CAD build for the part. Positions are in the model's coordinates, mm. A direction names the side the tool comes from. Coordinates: 2 decimals unless noted, no trailing zeros. Write each loop counter-clockwise with the first axis right and the second up, starting at its lowest first coordinate (ties: lowest second). Pieces come first, ordered by that corner, then holes. Notation, with made-up numbers: (-3, -32) -> (16, -32) arc R30 ccw to (16, -6) -> close; hole circle Ø8 at (18.5, 32.5). An arc over 180 degrees is marked (long way). Answer as CSV lines item,"result". Start each with the question number.
```python
from build123d import *

# Parameters (mm, degrees)
SKIZZE1_W                       = 60
SKIZZE1_H                       = 72.2
AUFSATZ_LINEAR_AUSTRAGEN1_DEPTH = 4
AUFSATZ_LINEAR_START            = -6
SKIZZE2_W                       = 60
SKIZZE2_H                       = 3
AUFSATZ_LINEAR_AUSTRAGEN2_DEPTH = 10
SKIZZE4_R                       = 2
SCHNITT_LINEAR_AUSTRAGEN1_DEPTH = 51.287274732
F_LLMUSTER1_OUTLINE_R           = 2
F_LLMUSTER1_DEPTH               = 4


# Read off the part's stored shape, not the designer's step: Füllmuster1
with BuildPart() as part:
    # Skizze1 → Aufsatz-Linear austragen1 (new body)
    with BuildSketch(Plane(origin=(0, 0, 0), x_dir=(1, 0, 0), z_dir=(0, 1, 0))):
        Rectangle(SKIZZE1_W, SKIZZE1_H)
    extrude(amount=AUFSATZ_LINEAR_AUSTRAGEN1_DEPTH)

    # Skizze2 → Aufsatz-Linear austragen2 (add)
    with BuildSketch(Plane(origin=(0, 0, 0), x_dir=(1, 0, 0), z_dir=(0, 1, 0)).offset(AUFSATZ_LINEAR_START)):
        with Locations((0, 37.6)):
            Rectangle(SKIZZE2_W, SKIZZE2_H)
    aufsatz_linear_austragen2 = extrude(amount=AUFSATZ_LINEAR_AUSTRAGEN2_DEPTH)

    # Spiegeln1: Aufsatz-Linear austragen2 across plane
    add(aufsatz_linear_austragen2.mirror(Plane.XY))

    # Skizze4 → Schnitt-Linear austragen1 (cut, through all)
    with BuildSketch(Plane(origin=(0, 4, 0), x_dir=(1, 0, 0), z_dir=(0, 1, 0))):
        with Locations(Location((0, 0, 0), (0, 0, 270))):
            Circle(SKIZZE4_R)
    extrude(amount=-SCHNITT_LINEAR_AUSTRAGEN1_DEPTH, mode=Mode.SUBTRACT)

    # Füllmuster1 outline → Füllmuster1 (cut)
    with BuildSketch(Plane(origin=(0, 0, 0), x_dir=(1, 0, 0), z_dir=(0, 1, 0))):
        with Locations((6.3, 0)):
            Circle(F_LLMUSTER1_OUTLINE_R)
        with Locations((17.760190533, 6.464180709)):
            Circle(F_LLMUSTER1_OUTLINE_R)
        with Locations((14.478239975, 12.148685823)):
            Circle(F_LLMUSTER1_OUTLINE_R)
        with Locations((9.45, 16.367880132)):
            Circle(F_LLMUSTER1_OUTLINE_R)
        with Locations((6.3, 10.911920088)):
            Circle(F_LLMUSTER1_OUTLINE_R)
        with Locations((0, 12.6)):
            Circle(F_LLMUSTER1_OUTLINE_R)
        with Locations((-6.3, 10.911920088)):
            Circle(F_LLMUSTER1_OUTLINE_R)
        with Locations((-10.911920088, 6.3)):
            Circle(F_LLMUSTER1_OUTLINE_R)
        with Locations((-12.6, 0)):
            Circle(F_LLMUSTER1_OUTLINE_R)
        with Locations((-10.911920088, -6.3)):
            Circle(F_LLMUSTER1_OUTLINE_R)
        with Locations((-6.3, -10.911920088)):
            Circle(F_LLMUSTER1_OUTLINE_R)
        with Locations((0, -12.6)):
            Circle(F_LLMUSTER1_OUTLINE_R)
        with Locations((3.15, -5.455960044)):
            Circle(F_LLMUSTER1_OUTLINE_R)
        with Locations((-3.15, -5.455960044)):
            Circle(F_LLMUSTER1_OUTLINE_R)
        with Locations((-6.3, 0)):
            Circle(F_LLMUSTER1_OUTLINE_R)
        with Locations((-3.15, 5.455960044)):
            Circle(F_LLMUSTER1_OUTLINE_R)
        with Locations((3.15, 5.455960044)):
            Circle(F_LLMUSTER1_OUTLINE_R)
        with Locations((12.6, 0)):
            Circle(F_LLMUSTER1_OUTLINE_R)
        with Locations((10.911920088, -6.3)):
            Circle(F_LLMUSTER1_OUTLINE_R)
        with Locations((6.3, -10.911920088)):
            Circle(F_LLMUSTER1_OUTLINE_R)
        with Locations((3.281950558, 18.612866532)):
            Circle(F_LLMUSTER1_OUTLINE_R)
        with Locations((-3.281950558, 18.612866532)):
            Circle(F_LLMUSTER1_OUTLINE_R)
        with Locations((-9.45, 16.367880132)):
            Circle(F_LLMUSTER1_OUTLINE_R)
        with Locations((-14.478239975, 12.148685823)):
            Circle(F_LLMUSTER1_OUTLINE_R)
        with Locations((-17.760190533, 6.464180709)):
            Circle(F_LLMUSTER1_OUTLINE_R)
        with Locations((-18.9, 0)):
            Circle(F_LLMUSTER1_OUTLINE_R)
        with Locations((-17.760190533, -6.464180709)):
            Circle(F_LLMUSTER1_OUTLINE_R)
        with Locations((-14.478239975, -12.148685823)):
            Circle(F_LLMUSTER1_OUTLINE_R)
        with Locations((-9.45, -16.367880132)):
            Circle(F_LLMUSTER1_OUTLINE_R)
        with Locations((-3.281950558, -18.612866532)):
            Circle(F_LLMUSTER1_OUTLINE_R)
        with Locations((3.281950558, -18.612866532)):
            Circle(F_LLMUSTER1_OUTLINE_R)
        with Locations((9.45, -16.367880132)):
            Circle(F_LLMUSTER1_OUTLINE_R)
        with Locations((14.478239975, -12.148685823)):
            Circle(F_LLMUSTER1_OUTLINE_R)
        with Locations((17.760190533, -6.464180709)):
            Circle(F_LLMUSTER1_OUTLINE_R)
        with Locations((18.9, 0)):
            Circle(F_LLMUSTER1_OUTLINE_R)
        with Locations((10.911920088, 6.3)):
            Circle(F_LLMUSTER1_OUTLINE_R)
    extrude(amount=F_LLMUSTER1_DEPTH, mode=Mode.SUBTRACT)


solid = part.part
```
1. Wall check: line 1 (Z direction, x = 6.3, y = 1.85); line 2 (Z direction, x = -25.5, y = -4.5); line 3 (X direction, y = 3.5, z = 18). Give the ranges that are in metal, low to high.
2. Tool access for faces 1 (the face through (0, 0, -9)), 2 (the face through (-7.542, 1.972, -16.969)): list every direction of +Z, -Z, +X, -X, +Y, -Y with a clear straight run to the whole face (end or side of a thin tool).
3. Cut at C-C (y = -5). Give the cut face in (x, z).
4. Cut at D-D (x = 3). Give the cut face in (y, z), then the cut area to 3 significant figures.
5. Cut at A-A (z = 0). Count the separate pieces of the cut face and the enclosed holes in it, then the cut area to 3 significant figures.
6. Flat gauge pins, fed straight in: P1, Ø3, axis at x = -12.6, z = 0, coming from the +Y side; P2, Ø5, axis at x = 0, z = -12.6, coming from the -Y side. Where does each tip first touch, or does it go through?
7. Mould opens along Z. For faces 3 (the face through (-10.753, 1.972, 0.766)), 4 (the face through (0, -6, -38)), 5 (the face through (20.808, 1.972, -0.601)), 6 (the face through (0, -1, 39.1)) say: pulls with the +Z half, pulls with the -Z half, needs draft (parallel to the pull), parting line crosses it, or undercut.
8. Cut at B-B (x = -6.3). Give the cut face in (y, z).
Geometry check:
1,line 1,"-39.1 to -12.91, -8.91 to -2, 2 to 8.91, 12.91 to 39.1"
1,line 2,"-39.1 to -36.1, 36.1 to 39.1"
1,line 3,"-30 to -10.61, -8.29 to -5.19, -1.38 to 1.38, 5.19 to 8.29, 10.61 to 30"
2,face 1,"+X, -X, -Y"
2,face 2,"+Y, -Y"
3,outline,"(-30, -39.1) -> (30, -39.1) -> (30, -36.1) -> (-30, -36.1) -> close; (-30, 36.1) -> (30, 36.1) -> (30, 39.1) -> (-30, 39.1) -> close"
4,outline,"(-6, -39.1) -> (4, -39.1) -> (4, -20.59) -> (0, -20.59) -> (0, -36.1) -> (-6, -36.1) -> close; (-6, 36.1) -> (0, 36.1) -> (0, 20.59) -> (4, 20.59) -> (4, 39.1) -> (-6, 39.1) -> close; (0, -16.63) -> (4, -16.63) -> (4, -7.45) -> (0, -7.45) -> close; (0, -3.46) -> (4, -3.46) -> (4, 3.46) -> (0, 3.46) -> close; (0, 7.45) -> (4, 7.45) -> (4, 16.63) -> (0, 16.63) -> close"
4,area,"285 mm²"
5,separate pieces,"8"
5,enclosed holes,"0"
5,area,"128 mm²"
6,P1,"through"
6,P2,"y = 0"
7,face 3,"undercut"
7,face 4,"needs draft"
7,face 5,"undercut"
7,face 6,"pulls with the +Z half"
8,outline,"(-6, -39.1) -> (4, -39.1) -> (4, -12.91) -> (0, -12.91) -> (0, -36.1) -> (-6, -36.1) -> close; (-6, 36.1) -> (0, 36.1) -> (0, 12.91) -> (4, 12.91) -> (4, 39.1) -> (-6, 39.1) -> close; (0, -8.91) -> (4, -8.91) -> (4, -2) -> (0, -2) -> close; (0, 2) -> (4, 2) -> (4, 8.91) -> (0, 8.91) -> close"
